Source: CAD feature listing. Evaluate the final solid. Frame: model axes, mm. Face numbers are marked on the shaded views. Coordinates: 2 decimals unless noted, no trailing zeros. Loops run counter-clockwise (first coordinate to the right, second up) from the corner with the lowest first, then second, coordinate; pieces in that order, holes last.
Item 1: Pull-direction query (X, two-part tool) for the marked faces 1 and 2; classes: +X half, -X half, draft (parallel to the pull), parting line (faces both ways), or undercut.
Item 2: Line query: probe 1 along Y at (x, z) = (0, 4.8); probe 2 along X at (y, z) = (-9.5, -0.5); probe 3 along X at (y, z) = (12.5, 5.5). Output: solid intervals per line, ascending.
Item 3: Section query A-A, the plane y = 0. Return the cut outline in (x, z), then the cut area to 3 significant figures.
Item 4: Section query B-B, the plane x = 0. State how many separate pieces and enclosed holes the cut face has, then the cut area to 3 significant figures.
Item 5: Pin query (flat end, axial travel): pin 1 Ø9.5 at (x, y) = (-21.75, 29.93) entering from +Z; pin 2 Ø2 at (y, z) = (5.5, 3.5) entering from +X; pin 3 Ø3 at (y, z) = (-21, 4) entering from -X; pin 4 Ø1.8 at (x, y) = (20.5, 28.5) entering from -Z. Return the tip coordinate at first contact, or that it passes through.
```python
from build123d import *

# Parameters (mm, degrees)
ESQUISSE1_R             = 42
ESQUISSE1_R_2           = 31.2
BOSS_EXTRU_1_DEPTH      = 6
BOSS_EXTRU_2_START      = 1
ESQUISSE2_R             = 42
ESQUISSE2_R_2           = 28.6
BOSS_EXTRU_2_DEPTH      = 1
ESQUISSE5_R             = 1.7
ENL_V_MAT_EXTRU_1_DEPTH = 60.808026217
ESQUISSE6_R             = 3
ENL_V_MAT_EXTRU_2_DEPTH = 3.2
CHANFREIN1_SIZE         = 0.6
CONG_2_R                = 1


with BuildPart() as part:
    # Esquisse1 → Boss.-Extru.1 (new body)
    with BuildSketch(Plane.XY):
        Circle(ESQUISSE1_R)
        Circle(ESQUISSE1_R_2, mode=Mode.SUBTRACT)
    extrude(amount=BOSS_EXTRU_1_DEPTH)

    # Esquisse2 → Boss.-Extru.2 (add)
    with BuildSketch(Plane(origin=(0, 0, 0), x_dir=(-1, 0, 0), z_dir=(0, 0, -1)).offset(BOSS_EXTRU_2_START)):
        Circle(ESQUISSE2_R)
        Circle(ESQUISSE2_R_2, mode=Mode.SUBTRACT)
    extrude(amount=-BOSS_EXTRU_2_DEPTH)

    # Esquisse5 → Enlèv. mat.-Extru.1 (cut, through all)
    with BuildSketch(Plane(origin=(0, 0, -1), x_dir=(-1, 0, 0), z_dir=(0, 0, -1))):
        with Locations((0, 37)):
            Circle(ESQUISSE5_R)
        with Locations((21.748054335, 29.933628792)):
            Circle(ESQUISSE5_R)
        with Locations((35.189091103, 11.433628792)):
            Circle(ESQUISSE5_R)
        with Locations((35.189091103, -11.433628792)):
            Circle(ESQUISSE5_R)
        with Locations((21.748054335, -29.933628792)):
            Circle(ESQUISSE5_R)
        with Locations((0, -37)):
            Circle(ESQUISSE5_R)
        with Locations((-21.748054335, -29.933628792)):
            Circle(ESQUISSE5_R)
        with Locations((-35.189091103, -11.433628792)):
            Circle(ESQUISSE5_R)
        with Locations((-35.189091103, 11.433628792)):
            Circle(ESQUISSE5_R)
        with Locations((-21.748054335, 29.933628792)):
            Circle(ESQUISSE5_R)
    extrude(amount=-ENL_V_MAT_EXTRU_1_DEPTH, mode=Mode.SUBTRACT)

    # Esquisse6 → Enlèv. mat.-Extru.2 (cut)
    with BuildSketch(Plane(origin=(0, 0, -1), x_dir=(-1, 0, 0), z_dir=(0, 0, -1))):
        with Locations((0, 37)):
            Circle(ESQUISSE6_R)
        with Locations((21.748054335, 29.933628792)):
            Circle(ESQUISSE6_R)
        with Locations((35.189091103, 11.433628792)):
            Circle(ESQUISSE6_R)
        with Locations((35.189091103, -11.433628792)):
            Circle(ESQUISSE6_R)
        with Locations((21.748054335, -29.933628792)):
            Circle(ESQUISSE6_R)
        with Locations((0, -37)):
            Circle(ESQUISSE6_R)
        with Locations((-21.748054335, -29.933628792)):
            Circle(ESQUISSE6_R)
        with Locations((-35.189091103, -11.433628792)):
            Circle(ESQUISSE6_R)
        with Locations((-35.189091103, 11.433628792)):
            Circle(ESQUISSE6_R)
        with Locations((-21.748054335, 29.933628792)):
            Circle(ESQUISSE6_R)
    extrude(amount=-ENL_V_MAT_EXTRU_2_DEPTH, mode=Mode.SUBTRACT)

    # Chanfrein1
    chanfrein1_edges = [part.edges().sort_by_distance(p)[0] for p in [
        (-31.2, 0, 6),
    ]]
    chamfer(chanfrein1_edges, length=CHANFREIN1_SIZE)

    # Congé2
    cong_2_edges = [part.edges().sort_by_distance(p)[0] for p in [
        (42, 0, -1),
    ]]
    fillet(cong_2_edges, radius=CONG_2_R - 0.0001)  # a hair under: the kernel refuses the full size


solid = part.part
```
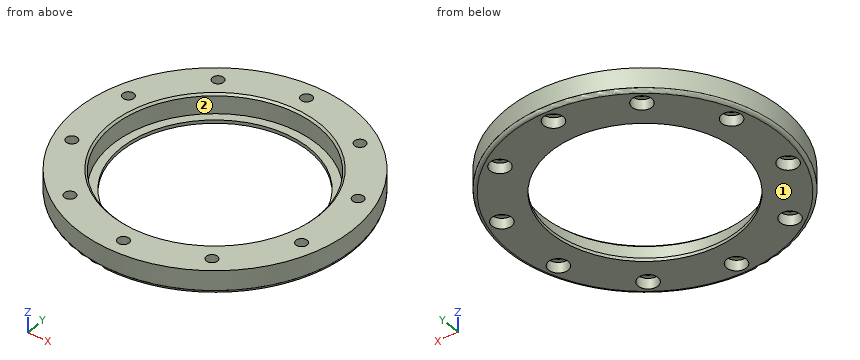
Verdict:
1. face 1: draft
1. face 2: undercut
2. probe 1: y = -42 to -38.7, -35.3 to -31.2, 31.2 to 35.3, 38.7 to 42
2. probe 2: x = -40.77 to -37.48, -32.9 to -26.98, 26.98 to 32.9, 37.48 to 40.77
2. probe 3: x = -40.1 to -36.51, -33.87 to -28.7, 28.7 to 33.87, 36.51 to 40.1
3. outline: (-42, 0) arc R1 ccw to (-41, -1) - (-28.6, -1) - (-28.6, 0) - (-31.2, 0) - (-31.2, 5.4) - (-31.8, 6) - (-42, 6) - close; (28.6, -1) - (41, -1) arc R1 ccw to (42, 0) - (42, 6) - (31.8, 6) - (31.2, 5.4) - (31.2, 0) - (28.6, 0) - close
3. area: 156 mm2
4. separate pieces: 4
4. enclosed holes: 0
4. area: 91.4 mm2
5. pin 1: stops at z = 6
5. pin 2: stops at x = 41.76
5. pin 3: stops at x = -37.2
5. pin 4: stops at z = 2.2
